Work out the finished part from the listing and answer in its coordinate system (mm). A direction names the side the tool comes from. Round coordinates to 2 decimals unless told otherwise and drop trailing zeros. Write each loop counter-clockwise with the first axis right and the second up, starting at its lowest first coordinate (ties: lowest second). Pieces come first, ordered by that corner, then holes. Notation, with made-up numbers: (-28, 29) -> (23, 29) arc R14 ccw to (23, 45) -> close; hole circle Ø8 at (-6.75, 81.25). An arc over 180 degrees is marked (long way). One line per item, written item: value.
```python
from build123d import *

# Parameters (mm, degrees)
F1_DEPTH = 5


with BuildPart() as f1:
    # F0 (on Top) → F1 (new body)
    with BuildSketch(Plane.XY):
        with BuildLine():
            Line((-171.635448, -70.591642), (-417.635441, -70.591642))
            Line((-417.635441, -70.591642), (-417.635441, -170.591642))
            Line((-417.635441, -170.591642), (-401.635441, -170.591642))
            Line((-401.635441, -170.591642), (-401.635441, -125.591642))
            ThreePointArc((-401.635441, -125.591642), (-392.635441, -116.591642), (-383.635441, -125.591642))
            Line((-383.635441, -125.591642), (-383.635441, -170.591642))
            Line((-383.635441, -170.591642), (-373.635441, -170.591642))
            Line((-373.635441, -170.591642), (-373.635441, -125.591642))
            ThreePointArc((-373.635441, -125.591642), (-364.635441, -116.591642), (-355.635441, -125.591642))
            Line((-355.635441, -125.591642), (-355.635441, -130.575008))
            Line((-355.635441, -130.575008), (-355.635441, -170.591642))
            Line((-355.635441, -170.591642), (-345.635441, -170.591642))
            Line((-345.635441, -170.591642), (-345.635441, -125.591642))
            ThreePointArc((-345.635441, -125.591642), (-336.643762, -116.583329), (-327.635448, -125.575008))
            Line((-327.635448, -125.575008), (-327.635448, -170.575008))
            Line((-327.635448, -170.575008), (-317.635448, -170.575008))
            Line((-317.635448, -170.575008), (-317.635448, -125.591642))
            ThreePointArc((-317.635448, -125.591642), (-308.635448, -116.591642), (-299.635448, -125.591642))
            Line((-299.635448, -125.591642), (-299.635448, -170.575008))
            Line((-299.635448, -170.575008), (-289.635448, -170.575008))
            Line((-289.635448, -170.575008), (-289.635448, -125.591642))
            ThreePointArc((-289.635448, -125.591642), (-280.635448, -116.591642), (-271.635448, -125.591642))
            Line((-271.635448, -125.591642), (-271.635448, -170.575008))
            Line((-271.635448, -170.575008), (-261.635448, -170.575008))
            Line((-261.635448, -170.575008), (-261.635448, -125.591642))
            ThreePointArc((-261.635448, -125.591642), (-252.635448, -116.591642), (-243.635448, -125.591642))
            Line((-243.635448, -125.591642), (-243.635448, -170.575008))
            Line((-243.635448, -170.575008), (-233.635448, -170.575008))
            Line((-233.635448, -170.575008), (-233.635448, -125.591642))
            ThreePointArc((-233.635448, -125.591642), (-224.635448, -116.591642), (-215.635448, -125.591642))
            Line((-215.635448, -125.591642), (-215.635448, -170.575008))
            Line((-215.635448, -170.575008), (-205.635448, -170.575008))
            Line((-205.635448, -170.575008), (-205.635448, -125.591642))
            ThreePointArc((-205.635448, -125.591642), (-196.635448, -116.591642), (-187.635448, -125.591642))
            Line((-187.635448, -125.591642), (-187.635448, -170.575008))
            Line((-187.635448, -170.575008), (-171.635448, -170.575008))
            Line((-171.635448, -170.575008), (-171.635448, -70.591642))
        make_face()
    extrude(amount=F1_DEPTH)


solid = f1.part
```
(1) Find section C-C on x = -252. Give the vertices of the cut face in (y, z).
Reported:
outline: (-116.61, 0) -> (-70.59, 0) -> (-70.59, 5) -> (-116.61, 5) -> close
(2) Find section A-A on y = -130. Give the number of separate pieces and of enclosed holes in the cut face, plus the area to 3 significant figures.
Reported:
separate pieces: 9
enclosed holes: 0
area: 510 mm2
(3) Consider probe 1 along Y at (x, z) = (-197, 2.45); probe 2 along Y at (x, z) = (-321, 0.8) (3 decimals). Determine where each line is inside the solid, lowest interval first.
Reported:
probe 1: y = -116.6 to -70.59
probe 2: y = -170.575 to -70.592
(4) A tool of negligible diameter and unlimited length cuts with its end or side. For faces 1 (the face through (-373.635, -148, 2)), 2 (the face through (-171.635, -121, 2)), from which of +Z, -Z, +X, -X, +Y, -Y can it reach the whole face along a straight path? Write none if from no direction.
Reported:
face 1: +Z, -Z, -Y
face 2: +Z, -Z, +X, +Y, -Y
(5) Find section B-B on x = -314.5. Give the vertices of the cut face in (y, z), plus the area to 3 significant figures.
Reported:
outline: (-118.76, 0) -> (-70.59, 0) -> (-70.59, 5) -> (-118.76, 5) -> close
area: 241 mm2
